```python
from build123d import *

# Parameters (mm, degrees)
SKETCH1_W           = 20.32
SKETCH1_H           = 41.91
BOSS_EXTRUDE1_DEPTH = 2.9972
SKETCH2_R           = 1.651
CUT_EXTRUDE1_DEPTH  = 35.793587165
CUT_EXTRUDE2_DEPTH  = 35.793587165
FILLET1_R           = 2.54


with BuildPart() as part:
    # Sketch1 → Boss-Extrude1 (new body)
    with BuildSketch(Plane.XY):
        with BuildLine():
            Line((16.51, 28.321), (5.334, 28.321))
            ThreePointArc((5.334, 28.321), (0, 30.48), (-5.334, 28.321))
            Line((-5.334, 28.321), (-16.51, 28.321))
            Line((-16.51, 28.321), (-16.51, -28.321))
            Line((-16.51, -28.321), (-5.334, -28.321))
            ThreePointArc((-5.334, -28.321), (0, -30.48), (5.334, -28.321))
            Line((5.334, -28.321), (16.51, -28.321))
            Line((16.51, -28.321), (16.51, 28.321))
        make_face()
        Rectangle(SKETCH1_W, SKETCH1_H, mode=Mode.SUBTRACT)
    extrude(amount=BOSS_EXTRUDE1_DEPTH)

    # Sketch2 → Cut-Extrude1 (cut, through all)
    with BuildSketch(Plane.XY.offset(2.9972)):
        with Locations((-5.08, 24)):
            Circle(SKETCH2_R)
        with Locations((5.08, 24)):
            Circle(SKETCH2_R)
        with Locations((5.08, -24)):
            Circle(SKETCH2_R)
        with Locations((-5.08, -24)):
            Circle(SKETCH2_R)
        with BuildLine():
            Line((-6.35, 20.955), (-6.35, -20.955))
            ThreePointArc((-6.35, -20.955), (-8.255, -22.86), (-10.16, -20.955))
            Line((-10.16, -20.955), (-10.16, 20.955))
            ThreePointArc((-10.16, 20.955), (-8.255, 22.86), (-6.35, 20.955))
        make_face()
        with BuildLine():
            Line((6.35, 20.955), (6.35, -20.955))
            ThreePointArc((6.35, -20.955), (8.255, -22.86), (10.16, -20.955))
            Line((10.16, -20.955), (10.16, 20.955))
            ThreePointArc((10.16, 20.955), (8.255, 22.86), (6.35, 20.955))
        make_face()
        with BuildLine():
            Line((-2.54, -24), (-2.54, 24))
            ThreePointArc((-2.54, 24), (0, 26.54), (2.54, 24))
            Line((2.54, 24), (2.54, -24))
            ThreePointArc((2.54, -24), (0, -26.54), (-2.54, -24))
        make_face()
    extrude(amount=-CUT_EXTRUDE1_DEPTH, mode=Mode.SUBTRACT)

    # Sketch3 → Cut-Extrude2 (cut, through all)
    with BuildSketch(Plane.XY.offset(2.9972)):
        with BuildLine():
            Line((-11.4935, 23.604394695), (-11.4935, 22.369605305))
            ThreePointArc((-11.4935, 22.369605305), (-13.335, 20.528105305), (-15.1765, 22.369605305))
            Line((-15.1765, 22.369605305), (-15.1765, 23.604394695))
            ThreePointArc((-15.1765, 23.604394695), (-13.335, 25.445894695), (-11.4935, 23.604394695))
        make_face()
        with BuildLine():
            Line((-11.4935, 15.730394695), (-11.4935, 14.495605305))
            ThreePointArc((-11.4935, 14.495605305), (-13.335, 12.654105305), (-15.1765, 14.495605305))
            Line((-15.1765, 14.495605305), (-15.1765, 15.730394695))
            ThreePointArc((-15.1765, 15.730394695), (-13.335, 17.571894695), (-11.4935, 15.730394695))
        make_face()
        with BuildLine():
            Line((-11.4935, 4.554394695), (-11.4935, 3.319605305))
            ThreePointArc((-11.4935, 3.319605305), (-13.335, 1.478105305), (-15.1765, 3.319605305))
            Line((-15.1765, 3.319605305), (-15.1765, 4.554394695))
            ThreePointArc((-15.1765, 4.554394695), (-13.335, 6.395894695), (-11.4935, 4.554394695))
        make_face()
        with BuildLine():
            Line((-11.4935, -3.319605305), (-11.4935, -4.554394695))
            ThreePointArc((-11.4935, -4.554394695), (-13.335, -6.395894695), (-15.1765, -4.554394695))
            Line((-15.1765, -4.554394695), (-15.1765, -3.319605305))
            ThreePointArc((-15.1765, -3.319605305), (-13.335, -1.478105305), (-11.4935, -3.319605305))
        make_face()
        with BuildLine():
            Line((-11.4935, -14.495605305), (-11.4935, -15.730394695))
            ThreePointArc((-11.4935, -15.730394695), (-13.335, -17.571894695), (-15.1765, -15.730394695))
            Line((-15.1765, -15.730394695), (-15.1765, -14.495605305))
            ThreePointArc((-15.1765, -14.495605305), (-13.335, -12.654105305), (-11.4935, -14.495605305))
        make_face()
        with BuildLine():
            Line((-11.4935, -22.369605305), (-11.4935, -23.604394695))
            ThreePointArc((-11.4935, -23.604394695), (-13.335, -25.445894695), (-15.1765, -23.604394695))
            Line((-15.1765, -23.604394695), (-15.1765, -22.369605305))
            ThreePointArc((-15.1765, -22.369605305), (-13.335, -20.528105305), (-11.4935, -22.369605305))
        make_face()
    cut_extrude2 = extrude(amount=-CUT_EXTRUDE2_DEPTH, mode=Mode.SUBTRACT)

    # Mirror1: Cut-Extrude2 across plane
    add(cut_extrude2.mirror(Plane(origin=(0, 0, 0), x_dir=(0, 0, 1), z_dir=(1, 0, 0))), mode=Mode.SUBTRACT)

    # Fillet1
    fillet1_edges = [part.edges().sort_by_distance(p)[0] for p in [
        (-16.51, -28.321, 1.4986),
        (-16.51, 28.321, 1.4986),
        (16.51, 28.321, 1.4986),
        (16.51, -28.321, 1.4986),
    ]]
    fillet(fillet1_edges, radius=FILLET1_R)


solid = part.part
```
Input: part model. Units: mm. Frame: model coordinates. A direction names the side the tool comes from. Round coordinates to 2 decimals unless told otherwise and drop trailing zeros. Loops run counter-clockwise (first coordinate to the right, second up) from the corner with the lowest first, then second, coordinate; pieces in that order, holes last. Notation, with made-up numbers: (69, -16.75) -> (92, -16.75) arc R13 ccw to (92, 4.25) -> close; hole circle Ø9 at (80, 20.5). An arc over 180 degrees is marked (long way). Write each question's results on one line, items separated by ' | '.
1. First-contact query: P1, Ø1.5, axis at x = 5, z = 2.5, coming from the -Y side; P2, Ø0.9, axis at x = -10, z = 1.5, coming from the -Y side; P3, Ø3, axis at x = 5.08, y = -24, coming from the -Z side. Flat tips, straight axial feed; report the tip coordinate or a pass-through.
Geometry results:
P1: y = -29.19 | P2: y = -28.32 | P3: through
2. Section D-D (z = 1.1). State how many separate pieces and enclosed holes the cut face has, and give its area (3 significant figures).
Geometry results:
separate pieces: 1 | enclosed holes: 17 | area: 754 mm2
3. Section B-B (y = 13.5). Return loops of the section in (x, z), and give its area (3 significant figures).
Geometry results:
outline: (-16.51, 0) -> (-14.88, 0) -> (-14.88, 3) -> (-16.51, 3) -> close; (-11.79, 0) -> (-10.16, 0) -> (-10.16, 3) -> (-11.79, 3) -> close; (10.16, 0) -> (11.79, 0) -> (11.79, 3) -> (10.16, 3) -> close; (14.88, 0) -> (16.51, 0) -> (16.51, 3) -> (14.88, 3) -> close | area: 19.5 mm2
4. Mould query, pull axis X, two halves, no side actions, for faces 1 (the face through (-0.08, -30.48, 1.48)), 2 (the face through (13.38, 17.57, 1.52)), 3 (the face through (15.176, -4, 2)), 4 (the face through (-10, 28.321, 1)). Classes: +X half, -X half, draft (parallel to the pull), parting line (faces both ways), or undercut.
Geometry results:
face 1: parting line | face 2: undercut | face 3: undercut | face 4: draft
5. Section C-C (x = 4). Return loops of the section in (y, z) (3 decimals), and give its area (3 significant figures).
Geometry results:
outline: (-29.354, 0) -> (-25.249, 0) -> (-25.249, 2.997) -> (-29.354, 2.997) -> close; (-22.751, 0) -> (-20.955, 0) -> (-20.955, 2.997) -> (-22.751, 2.997) -> close; (20.955, 0) -> (22.751, 0) -> (22.751, 2.997) -> (20.955, 2.997) -> close; (25.249, 0) -> (29.354, 0) -> (29.354, 2.997) -> (25.249, 2.997) -> close | area: 35.4 mm2
6. Set-up query: faces 5 (the face through (-13.295, -25.445, 1.52)), 6 (the face through (0.08, 30.48, 1.48)). Return all of +Z, -Z, +X, -X, +Y, -Y with unobstructed straight access to the full face (end or side cutting, diameter ignored); none if empty.
Geometry results:
face 5: +Z, -Z | face 6: +Z, -Z, +Y
7. Ray query, line 1 (X direction, y = -11, z = 1.35); line 2 (X direction, y = 22, z = 2.9); line 3 (Y direction, x = -5.08, z = 1.95) (3 decimals). Return the intervals inside material, ascending. Write a range as from..to.
Geometry results:
line 1: -16.51..-10.16, 10.16..16.51 | line 2: -16.51..-15.14, -11.53..-9.85, -6.66..-2.54, 2.54..6.66, 9.85..11.53, 15.14..16.51 | line 3: -28.556..-25.651, -22.349..-20.955, 20.955..22.349, 25.651..28.556
8. Section A-A (x = 0). Return loops of the section in (y, z).
Geometry results:
outline: (-30.48, 0) -> (-26.54, 0) -> (-26.54, 3) -> (-30.48, 3) -> close; (26.54, 0) -> (30.48, 0) -> (30.48, 3) -> (26.54, 3) -> close
